Check sheet for the modelled part. Datum: model origin and axes. Units: mm. Coordinates: 2 decimals unless noted, no trailing zeros. Write each loop counter-clockwise with the first axis right and the second up, starting at its lowest first coordinate (ties: lowest second). Pieces come first, ordered by that corner, then holes. Notation, with made-up numbers: (17.5, 79) -> (69.5, 79) arc R23 ccw to (69.5, 112) -> close; hole circle Ø8 at (39.25, -36). An arc over 180 degrees is marked (long way). Put each result on its own line as item: value.
```python
from build123d import *

# Parameters (mm, degrees)
Y_KSEKLIK_EKSTR_ZYON1_DEPTH = 2
RADYUS1_R                   = 1


with BuildPart() as part:
    # Çizim1 → Yükseklik-Ekstrüzyon1 (new body)
    with BuildSketch(Plane.XY):
        Polygon((0, -8.75), (0, 8.75), (6.495190528, 5), (6.495190528, -5), align=None)
    extrude(amount=Y_KSEKLIK_EKSTR_ZYON1_DEPTH)

    # Radyus1
    radyus1_edges = [part.edges().sort_by_distance(p)[0] for p in [
        (0, -8.75, 1),
        (0, 8.75, 1),
        (6.495190528, 5, 1),
        (6.495190528, -5, 1),
    ]]
    fillet(radyus1_edges, radius=RADYUS1_R)


solid = part.part
```
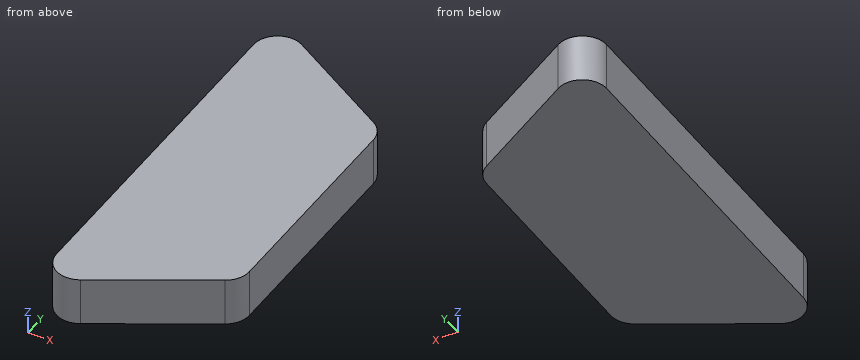
Q1. Cross-section at C-C (y = -6.25). Record the cut outline in (x, z).
Recorded:
outline: (0, 0) -> (4.33, 0) -> (4.33, 2) -> (0, 2) -> close
Q2. Cross-section at A-A (z = 0.45). Record the cut outline in (x, y), plus the area to 3 significant figures.
Recorded:
outline: (0, -7.02) arc R1 ccw to (1.5, -7.88) -> (6, -5.29) arc R1 ccw to (6.5, -4.42) -> (6.5, 4.42) arc R1 ccw to (6, 5.29) -> (1.5, 7.88) arc R1 ccw to (0, 7.02) -> close
area: 87.8 mm2
Q3. Material ranges on line 1 along X through (y, z) = (-4.5, 1.5); line 2 along Y through (x, z) = (2, 1.3); line 3 along Y through (x, z) = (2.5, 0.4), recorded low to high.
Recorded:
line 1: x = 0 to 6.49
line 2: y = -7.6 to 7.6
line 3: y = -7.31 to 7.31
Q4. Cross-section at B-B (x = 3.75). Record the cut outline in (y, z), plus the area to 3 significant figures.
Recorded:
outline: (-6.58, 0) -> (6.58, 0) -> (6.58, 2) -> (-6.58, 2) -> close
area: 26.3 mm2
